Geometry: final body of the model. Coordinates: model frame, mm. Round coordinates to 2 decimals unless told otherwise and drop trailing zeros. Write each loop counter-clockwise with the first axis right and the second up, starting at its lowest first coordinate (ties: lowest second). Pieces come first, ordered by that corner, then holes. Notation, with made-up numbers: M 64,38 L 94,38 A9 cw 94,54 Z; hole C 14,63 d2. An arc over 180 degrees is marked long. Use one line per item in the form item = value. Start each with the question number.
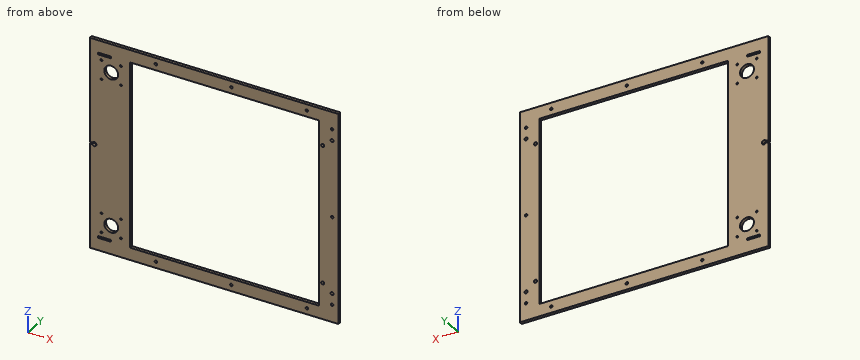
from build123d import *

# Parameters (mm, degrees)
SKETCH1_9_W         = 21
SKETCH1_9_H         = 3
SKETCH1_9_R         = 1.5
SKETCH1_9_R_2       = 11
SKETCH1_9_R_3       = 2
SKETCH1_9_R_4       = 2.5
SKETCH1_9_W_2       = 300
SKETCH1_9_H_2       = 300
BOSS_EXTRUDE7_DEPTH = 5


with BuildPart() as part:
    # Sketch1_9 → Boss-Extrude7 (new body)
    with BuildSketch(Plane(origin=(0, 0, 0), x_dir=(1, 0, 0), z_dir=(0, 1, 0))):
        with BuildLine():
            Line((-225, 170), (-225, 1.5))
            Line((-225, 1.5), (-221.16227766, 1.5))
            ThreePointArc((-221.16227766, 1.5), (-214.5, 0), (-221.16227766, -1.5))
            Line((-221.16227766, -1.5), (-225, -1.5))
            Line((-225, -1.5), (-225, -170))
            Line((-225, -170), (170, -170))
            Line((170, -170), (170, 170))
            Line((170, 170), (-225, 170))
        make_face()
        with Locations((-201.5, -148.5)):
            Rectangle(SKETCH1_9_W, SKETCH1_9_H, mode=Mode.SUBTRACT)
        with Locations(Location((-206.5, -139.5, 0), (0, 0, 270))):
            Circle(SKETCH1_9_R, mode=Mode.SUBTRACT)
        with Locations(Location((-191, -124, 0), (0, 0, 270))):
            Circle(SKETCH1_9_R_2, mode=Mode.SUBTRACT)
        with Locations(Location((-175.5, -139.5, 0), (0, 0, 270))):
            Circle(SKETCH1_9_R, mode=Mode.SUBTRACT)
        with Locations(Location((-120, -160, 0), (0, 0, 270))):
            Circle(SKETCH1_9_R_3, mode=Mode.SUBTRACT)
        with Locations(Location((-206.5, -108.5, 0), (0, 0, 270))):
            Circle(SKETCH1_9_R, mode=Mode.SUBTRACT)
        with Locations(Location((-175.5, -108.5, 0), (0, 0, 270))):
            Circle(SKETCH1_9_R, mode=Mode.SUBTRACT)
        with Locations(Location((0, -160, 0), (0, 0, 270))):
            Circle(SKETCH1_9_R_3, mode=Mode.SUBTRACT)
        with Locations(Location((120, -160, 0), (0, 0, 270))):
            Circle(SKETCH1_9_R_3, mode=Mode.SUBTRACT)
        with Locations(Location((160, -142, 0), (0, 0, 270))):
            Circle(SKETCH1_9_R_3, mode=Mode.SUBTRACT)
        with Locations(Location((160, -123.75, 0), (0, 0, 270))):
            Circle(SKETCH1_9_R_4, mode=Mode.SUBTRACT)
        with Locations(Location((145, -111.25, 0), (0, 0, 270))):
            Circle(SKETCH1_9_R_4, mode=Mode.SUBTRACT)
        with Locations(Location((-206.5, 108.5, 0), (0, 0, 270))):
            Circle(SKETCH1_9_R, mode=Mode.SUBTRACT)
        with Locations(Location((-175.5, 108.5, 0), (0, 0, 270))):
            Circle(SKETCH1_9_R, mode=Mode.SUBTRACT)
        with Locations(Location((-191, 124, 0), (0, 0, 270))):
            Circle(SKETCH1_9_R_2, mode=Mode.SUBTRACT)
        with Locations(Location((-206.5, 139.5, 0), (0, 0, 270))):
            Circle(SKETCH1_9_R, mode=Mode.SUBTRACT)
        with Locations(Location((-175.5, 139.5, 0), (0, 0, 270))):
            Circle(SKETCH1_9_R, mode=Mode.SUBTRACT)
        with Locations((-201.5, 148.5)):
            Rectangle(SKETCH1_9_W, SKETCH1_9_H, mode=Mode.SUBTRACT)
        with Locations(Location((-120, 160, 0), (0, 0, 270))):
            Circle(SKETCH1_9_R_3, mode=Mode.SUBTRACT)
        with Locations((-11, 0)):
            Rectangle(SKETCH1_9_W_2, SKETCH1_9_H_2, mode=Mode.SUBTRACT)
        with Locations(Location((160, 0, 0), (0, 0, 270))):
            Circle(SKETCH1_9_R_3, mode=Mode.SUBTRACT)
        with Locations(Location((0, 160, 0), (0, 0, 270))):
            Circle(SKETCH1_9_R_3, mode=Mode.SUBTRACT)
        with Locations(Location((145, 111.25, 0), (0, 0, 270))):
            Circle(SKETCH1_9_R_4, mode=Mode.SUBTRACT)
        with Locations(Location((160, 123.75, 0), (0, 0, 270))):
            Circle(SKETCH1_9_R_4, mode=Mode.SUBTRACT)
        with Locations(Location((120, 160, 0), (0, 0, 270))):
            Circle(SKETCH1_9_R_3, mode=Mode.SUBTRACT)
        with Locations(Location((160, 142, 0), (0, 0, 270))):
            Circle(SKETCH1_9_R_3, mode=Mode.SUBTRACT)
    extrude(amount=BOSS_EXTRUDE7_DEPTH)


solid = part.part
1. Section query C-C (y = 2.3). Give the number of separate pieces and of enclosed holes in the cut face, then the cut area to 3 significant figures.
2. Section query B-B (x = -15). Return loops of the section in (y, z), then the cut area to 3 significant figures.
3. Section query A-A (z = -72). Return loops of the section in (x, y), then the cut area to 3 significant figures.
4. Contact query for flat-ended pins moving along their axis: pin 1 (3 mm diameter, centred on x = -120, z = -160, fed in from +Y); pin 2 (6.5 mm diameter, centred on x = 160, z = -142, fed in from +Y). Output: stop coordinate, or through.
5. Ray query, probe 1 along Z at (x, y) = (-175.5, 2.85); probe 2 along X at (y, z) = (3.2, 108.5); probe 3 along X at (y, z) = (1.75, -142). Return the intervals inside material, ascending.
Checks:
q1.separate_pieces = 1
q1.enclosed_holes = 26
q1.area = 43,100 mm^2
q2.outline = M 0,-170 L 5,-170 L 5,-150 L 0,-150 Z; M 0,150 L 5,150 L 5,170 L 0,170 Z
q2.area = 200 mm^2
q3.outline = M -225,0 L -161,0 L -161,5 L -225,5 Z; M 139,0 L 170,0 L 170,5 L 139,5 Z
q3.area = 475 mm^2
q4.pin_1 = through
q4.pin_2 = 5
q5.probe_1 = -170 to -141, -138 to -110, -107 to 107, 110 to 138, 141 to 170
q5.probe_2 = -225 to -208, -205 to -177, -174 to -161, 139 to 170
q5.probe_3 = -225 to -161, 139 to 158, 162 to 170
